```python
from build123d import *

# Parameters (mm, degrees)
SKETCH4_W           = 70
SKETCH4_H           = 80
SKETCH4_R           = 2.5
BOSS_EXTRUDE2_DEPTH = 4
FILLET1_R           = 5
SKETCH6_R           = 1
SKETCH6_W           = 23
SKETCH6_H           = 12.5
CUT_EXTRUDE1_DEPTH  = 54.301031885


with BuildPart() as part:
    # Sketch4 → Boss-Extrude2 (new body)
    with BuildSketch(Plane.XY):
        Rectangle(SKETCH4_W, SKETCH4_H)
        with Locations((-27, 7)):
            Circle(SKETCH4_R, mode=Mode.SUBTRACT)
        with Locations(Location((27, 7, 0), (0, 0, 180))):
            Circle(SKETCH4_R, mode=Mode.SUBTRACT)
        with BuildLine():
            Line((-24.5, -34), (-24.5, -35))
            ThreePointArc((-24.5, -35), (-27, -37.5), (-29.5, -35))
            Line((-29.5, -35), (-29.5, -34))
            ThreePointArc((-29.5, -34), (-27, -31.5), (-24.5, -34))
        make_face(mode=Mode.SUBTRACT)
        with BuildLine():
            Line((24.5, -34), (24.5, -35))
            ThreePointArc((24.5, -35), (27, -37.5), (29.5, -35))
            Line((29.5, -35), (29.5, -34))
            ThreePointArc((29.5, -34), (27, -31.5), (24.5, -34))
        make_face(mode=Mode.SUBTRACT)
    extrude(amount=BOSS_EXTRUDE2_DEPTH)

    # Fillet1
    fillet1_edges = [part.edges().sort_by_distance(p)[0] for p in [
        (35, -40, 2),
        (-35, -40, 2),
        (-35, 40, 2),
        (35, 40, 2),
    ]]
    fillet(fillet1_edges, radius=FILLET1_R)

    # Sketch6 → Cut-Extrude1 (cut, through all)
    with BuildSketch(Plane.XY.offset(4)):
        with Locations((-13.75, -31)):
            Circle(SKETCH6_R)
        with Locations(Location((13.75, -31, 0), (0, 0, 180))):
            Circle(SKETCH6_R)
        with Locations((0, -31)):
            Rectangle(SKETCH6_W, SKETCH6_H)
        with BuildLine():
            Line((-6.5, 30), (-6.5, -10))
            ThreePointArc((-6.5, -10), (-8, -11.5), (-9.5, -10))
            Line((-9.5, -10), (-9.5, 30))
            ThreePointArc((-9.5, 30), (-8, 31.5), (-6.5, 30))
        make_face()
        with BuildLine():
            Line((6.5, 30), (6.5, -10))
            ThreePointArc((6.5, -10), (8, -11.5), (9.5, -10))
            Line((9.5, -10), (9.5, 30))
            ThreePointArc((9.5, 30), (8, 31.5), (6.5, 30))
        make_face()
    extrude(amount=-CUT_EXTRUDE1_DEPTH, mode=Mode.SUBTRACT)


solid = part.part
```
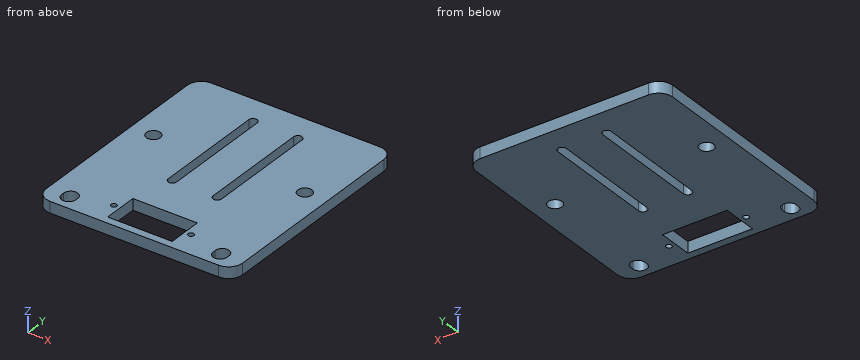
Work out the finished part from the listing and answer in its coordinate system (mm). Coordinates: 2 decimals unless noted, no trailing zeros. Order: outer loops, then holes, each group sorted by start corner. A loop starts at its lowest first (then second) coordinate and runs counter-clockwise, first axis right, second up. Notation, with made-up numbers: (36, 14.25) - (48, 14.25) arc R10 cw to (48, 20.25) - close; hole circle Ø5 at (5.25, 33.5). An arc over 180 degrees is marked (long way). Answer as a JSON object with one key per item and string values.
1. Find section D-D on z = 1.2. Count the separate pieces of the cut face and the enclosed holes in it, plus the area to 3 significant figures.
Output values:
{"separate pieces": "1", "enclosed holes": "9", "area": "4,940 mm²"}
2. Find section B-B on y = 23.5. Determine the outline of the cut face in (x, z).
Output values:
{"outline": "(-35, 0) - (-9.5, 0) - (-9.5, 4) - (-35, 4) - close; (-6.5, 0) - (6.5, 0) - (6.5, 4) - (-6.5, 4) - close; (9.5, 0) - (35, 0) - (35, 4) - (9.5, 4) - close"}
3. This flat-tipped pin is pushed along its axis until it touches: P1, Ø3, axis at x = 27, y = 7, coming from the -Z side. Where does it stop, or does it pass through?
Output values:
{"P1": "passes through"}
4. Find section C-C on x = 13.75. Determine the outline of the cut face in (y, z).
Output values:
{"outline": "(-40, 0) - (-32, 0) - (-32, 4) - (-40, 4) - close; (-30, 0) - (40, 0) - (40, 4) - (-30, 4) - close"}
5. Consider line 1 (Y direction, x = 27, z = 1.7); line 2 (Y direction, x = -8, z = 1.3); line 3 (X direction, y = 1, z = 1). Determine where each line is inside the solid, lowest interval first.
Output values:
{"line 1": "y = -40 to -37.5, -31.5 to 4.5, 9.5 to 40", "line 2": "y = -40 to -37.25, -24.75 to -11.5, 31.5 to 40", "line 3": "x = -35 to -9.5, -6.5 to 6.5, 9.5 to 35"}
6. Find section A-A on x = -8. Determine the outline of the cut face in (y, z), plus the area to 3 significant figures.
Output values:
{"outline": "(-40, 0) - (-37.25, 0) - (-37.25, 4) - (-40, 4) - close; (-24.75, 0) - (-11.5, 0) - (-11.5, 4) - (-24.75, 4) - close; (31.5, 0) - (40, 0) - (40, 4) - (31.5, 4) - close", "area": "98.0 mm²"}
